Input: part model. Units: mm. Frame: model coordinates. A direction names the side the tool comes from. Give positions to 0.01 mm unless a question says otherwise; leave off trailing zeros. Loops run counter-clockwise (first coordinate to the right, second up) from the corner with the lowest first, then second, coordinate; pieces in that order, holes last.
from build123d import *

# Parameters (mm, degrees)
SKETCH1_W            = 40
SKETCH1_H            = 20
BOSS_EXTRUDE1_DEPTH  = 40.4
SKETCH2_W            = 56.4
SKETCH2_H            = 20
BOSS_EXTRUDE2_DEPTH  = 3.175
CUT_EXTRUDE1_REACH   = 44.994
SKETCH3_R            = 2.5
CUT_EXTRUDE2_REACH   = 44.994
MIRROR2_COPY_1_REACH = 44.994
FILLET1_R            = 3
SKETCH5_W            = 6.5
SKETCH5_H            = 2
BOSS_EXTRUDE3_DEPTH  = 5
SKETCH6_R            = 2.921
BOSS_EXTRUDE4_DEPTH  = 5.08
SKETCH7_W            = 8.2
SKETCH7_H            = 1.651
BOSS_EXTRUDE5_DEPTH  = 1.905
CHAMFER1_SIZE        = 1.9
CHAMFER1_SIZE2       = 5.08
CHAMFER2_SIZE        = 5.08
CHAMFER2_SIZE2       = 1.9
SKETCH8_R            = 1.5
CUT_EXTRUDE3_DEPTH   = 9.25


with BuildPart() as part:
    # Sketch1 → Boss-Extrude1 (new body)
    with BuildSketch(Plane(origin=(0, 0, 0), x_dir=(1, 0, 0), z_dir=(0, 1, 0))):
        Rectangle(SKETCH1_W, SKETCH1_H)
    extrude(amount=BOSS_EXTRUDE1_DEPTH)

    # Sketch2 → Boss-Extrude2 (add)
    with BuildSketch(Plane(origin=(0, 27.7, 0), x_dir=(1, 0, 0), z_dir=(0, 1, 0))):
        Rectangle(SKETCH2_W, SKETCH2_H)
    extrude(amount=BOSS_EXTRUDE2_DEPTH)

    # Sketch3 → Cut-Extrude1 (cut, up to next)
    with BuildSketch(Plane(origin=(0, 30.875, 0), x_dir=(1, 0, 0), z_dir=(0, 1, 0)), mode=Mode.PRIVATE) as cut_extrude1_sk1:
        with Locations(Location((-24.75, 5, 0), (0, 0, 270))):
            Circle(SKETCH3_R)
    cut_extrude1_tool1 = extrude(cut_extrude1_sk1.sketch, amount=-CUT_EXTRUDE1_REACH, mode=Mode.PRIVATE) & part.part
    # Sketch3 → Cut-Extrude1 (cut, up to next)
    with BuildSketch(Plane(origin=(0, 30.875, 0), x_dir=(1, 0, 0), z_dir=(0, 1, 0)), mode=Mode.PRIVATE) as cut_extrude1_sk2:
        with Locations(Location((-24.75, -5, 0), (0, 0, 270))):
            Circle(SKETCH3_R)
    cut_extrude1_tool2 = extrude(cut_extrude1_sk2.sketch, amount=-CUT_EXTRUDE1_REACH, mode=Mode.PRIVATE) & part.part
    # Sketch3 → Cut-Extrude1 (cut, up to next)
    with BuildSketch(Plane(origin=(0, 30.875, 0), x_dir=(1, 0, 0), z_dir=(0, 1, 0)), mode=Mode.PRIVATE) as cut_extrude1_sk3:
        with Locations(Location((24.75, 5, 0), (0, 0, 270))):
            Circle(SKETCH3_R)
    cut_extrude1_tool3 = extrude(cut_extrude1_sk3.sketch, amount=-CUT_EXTRUDE1_REACH, mode=Mode.PRIVATE) & part.part
    # Sketch3 → Cut-Extrude1 (cut, up to next)
    with BuildSketch(Plane(origin=(0, 30.875, 0), x_dir=(1, 0, 0), z_dir=(0, 1, 0)), mode=Mode.PRIVATE) as cut_extrude1_sk4:
        with Locations(Location((24.75, -5, 0), (0, 0, 270))):
            Circle(SKETCH3_R)
    cut_extrude1_tool4 = extrude(cut_extrude1_sk4.sketch, amount=-CUT_EXTRUDE1_REACH, mode=Mode.PRIVATE) & part.part
    add(cut_extrude1_tool1.solids().sort_by_distance((-24.75, 30.875, -5))[0], mode=Mode.SUBTRACT)
    add(cut_extrude1_tool2.solids().sort_by_distance((-24.75, 30.875, 5))[0], mode=Mode.SUBTRACT)
    add(cut_extrude1_tool3.solids().sort_by_distance((24.75, 30.875, -5))[0], mode=Mode.SUBTRACT)
    add(cut_extrude1_tool4.solids().sort_by_distance((24.75, 30.875, 5))[0], mode=Mode.SUBTRACT)

    # Sketch4 → Cut-Extrude2 (cut, up to next)
    with BuildSketch(Plane(origin=(0, 30.875, 0), x_dir=(1, 0, 0), z_dir=(0, 1, 0)), mode=Mode.PRIVATE) as cut_extrude2_sk1:
        with BuildLine():
            Line((-27.041287847, -4), (-28.2, -4))
            Line((-28.2, -4), (-28.2, -6))
            Line((-28.2, -6), (-27.041287847, -6))
            ThreePointArc((-27.041287847, -6), (-27.25, -5), (-27.041287847, -4))
        make_face()
    cut_extrude2_tool1 = extrude(cut_extrude2_sk1.sketch, amount=-CUT_EXTRUDE2_REACH, mode=Mode.PRIVATE) & part.part
    cut_extrude2 = cut_extrude2_tool1.solids().sort_by_distance((-27.68894, 30.875, 5))[0]
    add(cut_extrude2, mode=Mode.SUBTRACT)

    # Mirror1: Cut-Extrude2 across plane
    add(cut_extrude2.mirror(Plane(origin=(0, 0, 0), x_dir=(0, 0, 1), z_dir=(1, 0, 0))), mode=Mode.SUBTRACT)

    # Mirror2: Cut-Extrude2 across plane
    add(cut_extrude2.mirror(Plane.XY), mode=Mode.SUBTRACT)

    # Mirror2 copy 1 sketch → Mirror2 copy 1 (cut, up to next)
    with BuildSketch(Plane(origin=(0, 30.875, 0), x_dir=(-1, 0, 0), z_dir=(0, 1, 0)), mode=Mode.PRIVATE) as mirror2_copy_1_sk1:
        with BuildLine():
            Line((-27.041287847, -4), (-28.2, -4))
            Line((-28.2, -4), (-28.2, -6))
            Line((-28.2, -6), (-27.041287847, -6))
            ThreePointArc((-27.041287847, -6), (-27.25, -5), (-27.041287847, -4))
        make_face()
    mirror2_copy_1_tool1 = extrude(mirror2_copy_1_sk1.sketch, amount=-MIRROR2_COPY_1_REACH, mode=Mode.PRIVATE) & part.part
    add(mirror2_copy_1_tool1.solids().sort_by_distance((27.68894, 30.875, -5))[0], mode=Mode.SUBTRACT)

    # Fillet1
    fillet1_edges = [part.edges().sort_by_distance(p)[0] for p in [
        (28.2, 29.2875, -10),
        (-28.2, 29.2875, 10),
        (28.2, 29.2875, 10),
        (-28.2, 29.2875, -10),
    ]]
    fillet(fillet1_edges, radius=FILLET1_R)

    # Sketch5 → Boss-Extrude3 (add)
    with BuildSketch(Plane(origin=(20, 0, 0), x_dir=(0, 0, -1), z_dir=(1, 0, 0))):
        with Locations((0, 4.75)):
            Rectangle(SKETCH5_W, SKETCH5_H)
    extrude(amount=BOSS_EXTRUDE3_DEPTH)

    # Sketch6 → Boss-Extrude4 (add)
    with BuildSketch(Plane(origin=(0, 40.4, 0), x_dir=(1, 0, 0), z_dir=(0, 1, 0))):
        with Locations(Location((9.464, 0, 0), (0, 0, 270))):
            Circle(SKETCH6_R)
    extrude(amount=BOSS_EXTRUDE4_DEPTH)

    # Sketch7 → Boss-Extrude5 (add)
    with BuildSketch(Plane(origin=(0, 30.875, 0), x_dir=(1, 0, 0), z_dir=(0, 1, 0))):
        with Locations((24.1, 0)):
            Rectangle(SKETCH7_W, SKETCH7_H)
    boss_extrude5 = extrude(amount=BOSS_EXTRUDE5_DEPTH)

    # Chamfer1
    chamfer1_edges = [part.edges().sort_by_distance(p)[0] for p in [
        (28.2, 32.78, 0),
    ]]
    chamfer1_side = [part.faces().sort_by_distance(p)[0] for p in [
        (28.2, 29.567361633, 0),
    ]]
    chamfer(chamfer1_edges, length=CHAMFER1_SIZE, length2=CHAMFER1_SIZE2, reference=chamfer1_side[0])

    # Mirror3: Boss-Extrude5 across plane
    add(boss_extrude5.mirror(Plane(origin=(0, 0, 0), x_dir=(0, 0, 1), z_dir=(1, 0, 0))))

    # Chamfer2
    chamfer2_edges = [part.edges().sort_by_distance(p)[0] for p in [
        (-28.2, 32.78, 0),
    ]]
    chamfer2_side = [part.faces().sort_by_distance(p)[0] for p in [
        (-24.1, 32.78, 0),
    ]]
    chamfer(chamfer2_edges, length=CHAMFER2_SIZE, length2=CHAMFER2_SIZE2, reference=chamfer2_side[0])

    # Sketch8 → Cut-Extrude3 (cut)
    with BuildSketch(Plane(origin=(0, 45.48, 0), x_dir=(1, 0, 0), z_dir=(0, 1, 0))):
        with Locations(Location((9.464, 0, 0), (0, 0, 270))):
            Circle(SKETCH8_R)
    extrude(amount=-CUT_EXTRUDE3_DEPTH, mode=Mode.SUBTRACT)


solid = part.part
(1) Cut plane B-B (z = 5). Return the cut outline in (x, y) (3 decimals).
Values follow:
outline: (-22.25, 27.7) - (-20, 27.7) - (-20, 0) - (20, 0) - (20, 27.7) - (22.25, 27.7) - (22.25, 30.875) - (20, 30.875) - (20, 40.4) - (-20, 40.4) - (-20, 30.875) - (-22.25, 30.875) - close
(2) Cut plane D-D (y = 35.5). Return the cut outline in (x, z), and give its area (3 significant figures).
Values follow:
outline: (-20, -10) - (20, -10) - (20, 10) - (-20, 10) - close
area: 800 mm2
(3) Pin query (flat end, axial travel): pin 1 Ø2.5 at (x, z) = (23.5, 0) entering from -Y; pin 2 Ø8 at (x, z) = (-24.75, 5) entering from -Y; pin 3 Ø6 at (x, z) = (-10, -0.5) entering from +Y; pin 4 Ø3 at (x, z) = (24.75, 5) entering from +Y. Return the tip coordinate at first contact, or that it passes through.
Values follow:
pin 1: stops at y = 3.75
pin 2: stops at y = 27.7
pin 3: stops at y = 40.4
pin 4: passes through
(4) Cut plane C-C (x = -13). Return the cut outline in (y, z).
Values follow:
outline: (0, -10) - (40.4, -10) - (40.4, 10) - (0, 10) - close
(5) Cut plane A-A (x = -24). Return the cut outline in (y, z) (1 decimal), and give its area (3 significant figures).
Values follow:
outline: (27.7, -10) - (30.9, -10) - (30.9, -7.4) - (27.7, -7.4) - close; (27.7, -2.6) - (30.9, -2.6) - (30.9, -0.8) - (32.5, -0.8) - (32.5, 0.8) - (30.9, 0.8) - (30.9, 2.6) - (27.7, 2.6) - close; (27.7, 7.4) - (30.9, 7.4) - (30.9, 10) - (27.7, 10) - close
area: 35.8 mm2
(6) Reachability of faces 4 (the flat face through (-23, 32, 0.826)), 5 (the flat face through (22, 30.875, 5)), 6 (the flat face through (-28, 29, -4)), 7 (the flat face through (22, 30.875, -5)), 8 (the flat face through (28, 29, 6)) from +Z, -Z, +X, -X, +Y, -Y: full face, straight path, thin tool, end or side. Return the list, or none.
Values follow:
face 4: +Z, -X, +Y
face 5: +Z, +X, +Y
face 6: -X, +Y, -Y
face 7: -Z, +X, +Y
face 8: +X, +Y, -Y
(7) Mould query, pull axis Y, two halves, no side actions, for faces 1 (the flat face through (22, 5.75, 0)), 2 (the flat face through (-22, 30.875, 6)), 3 (the flat face through (22, 5, -3.25)). Classes: +Y half, -Y half, draft (parallel to the pull), parting line (faces both ways), or undercut.
Values follow:
face 1: undercut
face 2: +Y half
face 3: draft
(8) Ray query, probe 1 along Z at (x, y) = (24.75, 29.35); probe 2 along Y at (x, z) = (21, 0.5); probe 3 along X at (y, z) = (27.5, -6). Return the intervals inside material, ascending.
Values follow:
probe 1: z = -10 to -7.5, -2.5 to 2.5, 7.5 to 10
probe 2: y = 3.75 to 5.75, 27.7 to 32.78
probe 3: x = -20 to 20
